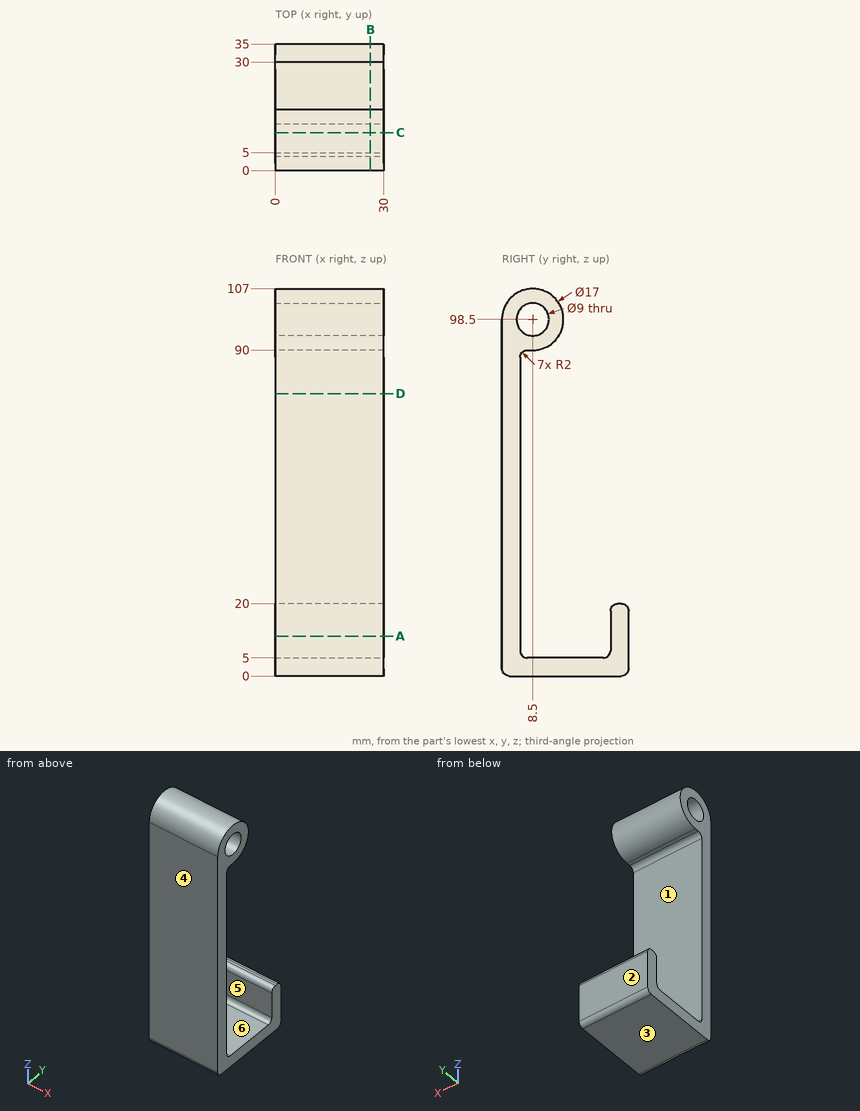
Here's the drawing with two shaded views (mm, measured from the low corner). I have some questions. A direction names the side the tool comes from. Coordinates: 2 decimals unless noted, no trailing zeros. Write each loop counter-clockwise with the first axis right and the second up, starting at its lowest first coordinate (ties: lowest second). Pieces come first, ordered by that corner, then holes. Notation, with made-up numbers: (-37, -9.75) -> (-15, -9.75) arc R18 ccw to (-15, -4.75) -> close; hole circle Ø7 at (19.25, 54.25). An arc over 180 degrees is marked (long way). Use a Markdown table: item, result. Add a question column.
(1) If we section it at C-C, the plane y = 10.5: Write out the boundary of the cut face in (x, z).
(2) If we section it at D-D, the plane z = 78: Write out the boundary of the cut face in (x, y), and give its area (3 significant figures).
(3) If we section it at B-B, the plane x = 26.25: Write out the boundary of the cut face in (y, z), and give its area (3 significant figures).
(4) I'm going to push flat-ended pins straight in: P1, Ø2, axis at x = 7.5, y = 31.5, coming from the +Z side; P2, Ø1.2, axis at x = 11.5, y = 7.5, coming from the -Z side; P3, Ø5.5, axis at y = 8.5, z = 98.5, coming from the +X side; P4, Ø1, axis at x = 26.5, z = 66.5, coming from the +Y side. Where does each tip first touch, or does it pass through?
(5) For the marked faces 4, 5 and 6, which set-ups out of +Z, -Z, +X, -X, +Y, -Y let a thin tool reach every point of the face, with its end or its side?
(6) Please list where these lines run through material, in increasing order: line 1 (Y direction, x = 13.5, z = 98.5); line 2 (Y direction, x = 12, z = 7.5); line 3 (Y direction, x = 9.75, z = 31).
(7) We'd pull the mould along Y, two halves only. Please class the marked faces 1, 2 and 3: +Y half, -Y half, draft (parallel to the pull), parting line (faces both ways), or undercut.
(8) If we section it at A-A, the plane z = 11: Write out the boundary of the cut face in (x, y), and give its area (3 significant figures).
Outcome:
| question | item | result |
|---|---|---|
| 1 | outline | (0, 0) -> (30, 0) -> (30, 5) -> (0, 5) -> close; (0, 90.24) -> (30, 90.24) -> (30, 94.47) -> (0, 94.47) -> close; (0, 102.53) -> (30, 102.53) -> (30, 106.76) -> (0, 106.76) -> close |
| 2 | outline | (0, 0) -> (30, 0) -> (30, 5) -> (0, 5) -> close |
| 2 | area | 150 mm^2 |
| 3 | outline | (0, 2) arc R2 ccw to (2, 0) -> (33, 0) arc R2 ccw to (35, 2) -> (35, 18) arc R2 ccw to (33, 20) -> (32, 20) arc R2 ccw to (30, 18) -> (30, 7) arc R2 cw to (28, 5) -> (7, 5) arc R2 cw to (5, 7) -> (5, 88) arc R2 cw to (7, 90) -> (8.5, 90) arc R8.5 ccw (long way) to (0, 98.5) -> close; hole circle Ø9 at (8.5, 98.5) |
| 3 | area | 853 mm^2 |
| 4 | P1 | stops at z = 20 |
| 4 | P2 | stops at z = 0 |
| 4 | P3 | passes through |
| 4 | P4 | stops at y = 5 |
| 5 | face 4 | +Z, -Z, +X, -X, -Y |
| 5 | face 5 | +Z, +X, -X |
| 5 | face 6 | +X, -X |
| 6 | line 1 | y = 0 to 4, 13 to 17 |
| 6 | line 2 | y = 0 to 5, 30 to 35 |
| 6 | line 3 | y = 0 to 5 |
| 7 | face 1 | undercut |
| 7 | face 2 | +Y half |
| 7 | face 3 | draft |
| 8 | outline | (0, 0) -> (30, 0) -> (30, 5) -> (0, 5) -> close; (0, 30) -> (30, 30) -> (30, 35) -> (0, 35) -> close |
| 8 | area | 300 mm^2 |
